Build history of the part. All positions in model axes, mm. Give positions to 0.01 mm unless a question says otherwise; leave off trailing zeros. Order: outer loops, then holes, each group sorted by start corner. A loop starts at its lowest first (then second) coordinate and runs counter-clockwise, first axis right, second up. Notation, with made-up numbers: (3, 59.25) -> (49, 59.25) arc R27 ccw to (49, 80.25) -> close; hole circle Ø8 at (-28, -20.75). An arc over 180 degrees is marked (long way). One line per question, with ' | ' between items. Start each with the question number.
(1) Drill centre lines: L1, parallel to Y at x = 7.5, z = 0.4; L2, parallel to Y at x = 20, z = 0.7; L3, parallel to X at y = 6.75, z = 1.05. Where is each one in solid material? Low to high. Write a range as from..to.
(2) Pin check, flat tip, straight feed: pin 1 Ø2.5 at (x, y) = (7.5, 5) entering from +Z. Stop position of the tip, or through.
(3) Cut at A-A (y = 5). Give the cut face in (x, z).
(4) Cut at C-C (z = 1.2). Give the cut face in (x, y), then the cut area to 3 significant figures.
(5) Cut at D-D (x = 7.5). Give the cut face in (y, z).
(6) Cut at B-B (x = 20). Give the cut face in (y, z), then the cut area to 3 significant figures.
from build123d import *

# Parameters (mm, degrees)
EXTRUSION1_DEPTH = 2
ESQUISSE2_R      = 1.5
EXTRUSION2_DEPTH = 48.212286536


with BuildPart() as part:
    # Esquisse1 → Extrusion1 (new body)
    with BuildSketch(Plane.XY):
        Polygon((0, 0), (15, 0), (40, 0), (40, 15), (15, 15), (15, 25), (0, 25), align=None)
    extrude(amount=EXTRUSION1_DEPTH)

    # Esquisse2 → Extrusion2 (cut, through all)
    with BuildSketch(Plane.XY.offset(2)):
        with Locations((7.5, 20)):
            Circle(ESQUISSE2_R)
        with Locations((7.5, 5)):
            Circle(ESQUISSE2_R)
        with Locations((20, 7.5)):
            Circle(ESQUISSE2_R)
        with Locations((35, 7.5)):
            Circle(ESQUISSE2_R)
    extrude(amount=-EXTRUSION2_DEPTH, mode=Mode.SUBTRACT)


solid = part.part
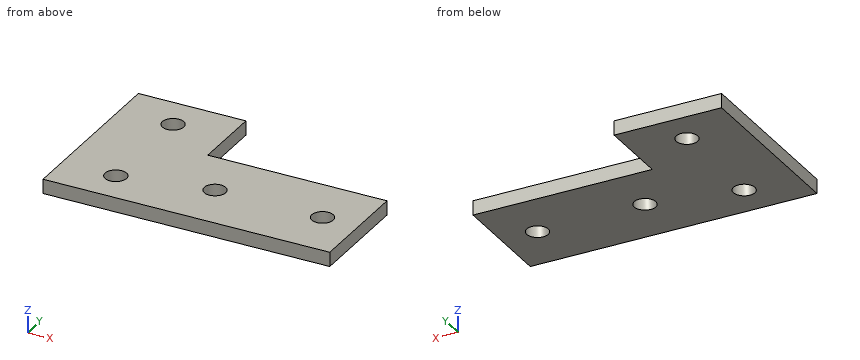
Result set:
1) L1: y = 0..3.5, 6.5..18.5, 21.5..25 | L2: y = 0..6, 9..15 | L3: x = 0..18.7, 21.3..33.7, 36.3..40
2) pin 1: passes through
3) outline: (0, 0) -> (6, 0) -> (6, 2) -> (0, 2) -> close; (9, 0) -> (40, 0) -> (40, 2) -> (9, 2) -> close
4) outline: (0, 0) -> (40, 0) -> (40, 15) -> (15, 15) -> (15, 25) -> (0, 25) -> close; hole circle Ø3 at (7.5, 5); hole circle Ø3 at (7.5, 20); hole circle Ø3 at (20, 7.5); hole circle Ø3 at (35, 7.5) | area: 722 mm2
5) outline: (0, 0) -> (3.5, 0) -> (3.5, 2) -> (0, 2) -> close; (6.5, 0) -> (18.5, 0) -> (18.5, 2) -> (6.5, 2) -> close; (21.5, 0) -> (25, 0) -> (25, 2) -> (21.5, 2) -> close
6) outline: (0, 0) -> (6, 0) -> (6, 2) -> (0, 2) -> close; (9, 0) -> (15, 0) -> (15, 2) -> (9, 2) -> close | area: 24.0 mm2
